```python
from build123d import *

# Parameters (mm, degrees)
F0_W     = 10
F0_H     = 40
F1_DEPTH = 16
F3_R     = 1.25
F4_DEPTH = 2.5
F5_R     = 0.5
F6_R     = 1
F7_SIZE  = 2
F8_R     = 1.6
F9_DEPTH = 10.001


with BuildPart() as f1:
    # F0 (on Top) → F1 (new body)
    with BuildSketch(Plane.XY):
        Rectangle(F0_W, F0_H)
    extrude(amount=F1_DEPTH)

    # F3 (on face) → F4 (join)
    with BuildSketch(Plane.XY.offset(16)):
        with Locations((0, 15.33)):
            Circle(F3_R)
    extrude(amount=F4_DEPTH)

    # F5
    f5_edges = [f1.edges().sort_by_distance(p)[0] for p in [
        (-1.25, 15.33, 18.5),
    ]]
    fillet(f5_edges, radius=F5_R)

    # F6
    f6_edges = [f1.edges().sort_by_distance(p)[0] for p in [
        (0, 20, 16),
        (0, 20, 0),
    ]]
    fillet(f6_edges, radius=F6_R)

    # F7
    f7_edges = [f1.edges().sort_by_distance(p)[0] for p in [
        (0, -20, 0),
        (0, -20, 16),
    ]]
    chamfer(f7_edges, length=F7_SIZE)

    # F8 (on face) → F9 (cut, through all)
    with BuildSketch(Plane(origin=(-5, 0, 0), x_dir=(0, -1, 0), z_dir=(-1, 0, 0))):
        with Locations((-17.05, 2.95)):
            Circle(F8_R)
        with Locations((4.95, 13.35)):
            Circle(F8_R)
    extrude(amount=-F9_DEPTH, mode=Mode.SUBTRACT)


solid = f1.part
```
Can you work these out from the model? Positions are in its coordinate system, mm. A direction names the side the tool comes from. Coordinates: 2 decimals unless noted, no trailing zeros. Write each loop counter-clockwise with the first axis right and the second up, starting at its lowest first coordinate (ties: lowest second). Pieces come first, ordered by that corner, then holes. Notation, with made-up numbers: M -27,79 L 2,79 A29 cw 2,117 Z; hole C -11,-37 d3. An arc over 180 degrees is marked long. Answer as CSV lines item,"result".
Item 1: Imagine slicing it at D-D on x = -3.5. List the corners of the cut face in (y, z) for me, plus the area to 3 significant figures.
Geometry results:
outline,"M -20,2 L -18,0 L 19,0 A1 ccw 20,1 L 20,15 A1 ccw 19,16 L -18,16 L -20,14 Z; hole C -4.95,13.35 d3.2; hole C 17.05,2.95 d3.2"
area,"619 mm2"
Item 2: We'd pull the mould along Z, two halves only. Please class faces 3 (the flat face through (0, -19, 15)), 4 (the cylindrical face through (-0.07, -6.476, 13.831)), 5 (the cylindrical face through (-0.07, 17.4, 1.39)), 6 (the flat face through (5, 0, 8)): +Z half, -Z half, draft (parallel to the pull), parting line (faces both ways), or undercut.
Geometry results:
face 3,"+Z half"
face 4,"undercut"
face 5,"undercut"
face 6,"draft"
Item 3: I'm going to push a flat-ended pin straight in: P1, Ø3.5, axis at y = -4.95, z = 13.35, coming from the -X side. Where does the tip first touch, or does it pass through?
Geometry results:
P1,"stops at x = -5"
Item 4: Imagine slicing it at C-C on x = 0. List the corners of the cut face in (y, z) for me.
Geometry results:
outline,"M -20,2 L -18,0 L 19,0 A1 ccw 20,1 L 20,15 A1 ccw 19,16 L 16.58,16 L 16.58,18 A0.5 ccw 16.08,18.5 L 14.58,18.5 A0.5 ccw 14.08,18 L 14.08,16 L -18,16 L -20,14 Z; hole C -4.95,13.35 d3.2; hole C 17.05,2.95 d3.2"
Item 5: Imagine slicing it at B-B on y = -4.95. List the corners of the cut face in (x, z) for me, plus the area to 3 significant figures.
Geometry results:
outline,"M -5,0 L 5,0 L 5,11.75 L -5,11.75 Z; M -5,14.95 L 5,14.95 L 5,16 L -5,16 Z"
area,"128 mm2"
Item 6: On a 3-axis mill with a long thin cutter (end or side, diameter ignored), from which of +Z, -Z, +X, -X, +Y, -Y can I reach the whole of each face in a straight line? I mean faces 1 (the cylindrical face through (-0.27, 14.11, 16.99)), 2 (the cylindrical face through (0.07, 19.715, 0.301)). Say none if no direction works.
Geometry results:
face 1,"+Z"
face 2,"-Z, +X, -X, +Y"
Item 7: Please list where these lines run through material, in increasing order: line 1 along Z through (x, y) = (-2.25, 17.05); line 2 along Z through (x, y) = (-1.75, -4.95); line 3 along Y through (x, z) = (-3.5, 13.25).
Geometry results:
line 1,"z = 0 to 1.35, 4.55 to 16"
line 2,"z = 0 to 11.75, 14.95 to 16"
line 3,"y = -20 to -6.55, -3.35 to 20"
Item 8: Imagine slicing it at A-A on z = 2.95. List the corners of the cut face in (x, y) for me.
Geometry results:
outline,"M -5,-20 L 5,-20 L 5,15.45 L -5,15.45 Z; M -5,18.65 L 5,18.65 L 5,20 L -5,20 Z"
